from build123d import *

# Parameters (mm, degrees)
F1_DEPTH = 63.5
F2_DEPTH = 25.4


with BuildPart() as f1:
    # F0 (on Front) → F1 (new body, symmetric)
    with BuildSketch(Plane.XZ):
        Polygon((22.225, 9.525), (-41.275, 9.525), (-41.275, -9.525), (41.275, -9.525), (41.275, 9.525), align=None)
    extrude(amount=F1_DEPTH, both=True)

    # F0 (on Front) → F2 (join, symmetric)
    with BuildSketch(Plane.XZ):
        with BuildLine():
            add(Edge.make_bspline(
                [(-41.275, 9.525), (-17.963025, 64.389196), (-0.915335, 58.434684), (52.727391, 61.644047)],
                knots=[0, 0, 0, 0, 108.575172, 108.575172, 108.575172, 108.575172], degree=3))
            Line((-41.275, 9.525), (22.225, 9.525))
            Line((22.225, 9.525), (22.225, 27.0002))
            ThreePointArc((22.225, 27.0002), (30.937262, 50.079368), (52.727391, 61.644047))
        make_face()
        with BuildLine():
            Line((22.225, 27.0002), (22.225, 9.525))
            Line((22.225, 9.525), (41.275, 9.525))
            Line((41.275, 9.525), (41.275, 27.0002))
            ThreePointArc((41.275, 27.0002), (45.92468, 38.22552), (57.15, 42.8752))
            Line((57.15, 42.8752), (60.325, 42.8752))
            Line((60.325, 42.8752), (60.325, 61.9252))
            Line((60.325, 61.9252), (57.15, 61.9252))
            add(Edge.make_bspline(
                [(52.727391, 61.644047), (54.174675, 61.730636), (55.648598, 61.823896), (57.15, 61.9252)],
                knots=[108.575172, 108.575172, 108.575172, 108.575172, 111.504536, 111.504536, 111.504536, 111.504536], degree=3))
            ThreePointArc((52.727391, 61.644047), (30.937262, 50.079368), (22.225, 27.0002))
        make_face()
    extrude(amount=F2_DEPTH, both=True)


solid = f1.part
The listing builds one solid part. Answer for the finished solid, in the listing's coordinates (mm). A direction names the side the tool comes from. Coordinates: 2 decimals unless noted, no trailing zeros. Order: outer loops, then holes, each group sorted by start corner. A loop starts at its lowest first (then second) coordinate and runs counter-clockwise, first axis right, second up. Notation, with made-up numbers: (18.5, -20) -> (43.5, -20) arc R20 ccw to (43.5, -2) -> close; hole circle Ø7 at (27, 2.25). An arc over 180 degrees is marked (long way). Answer in a Markdown table with one row per item. Add a question column.
Item 1: Each of these flat-tipped pins is pushed along its axis until it touches: P1, Ø8, axis at x = 41.5, z = 21.5, coming from the -Y side; P2, Ø1, axis at y = -8, z = 12, coming from the -X side; P3, Ø12, axis at x = -8.5, z = 25, coming from the +Y side. Where does it stop, or does it pass through?
Item 2: Find the intervals of material crossed by L1, parallel to Y at x = 2.5, z = 26; L2, parallel to Z at x = 9, y = 35.5 (3 decimals); L3, parallel to X at y = 12.5, z = -5 (3 decimals), in increasing order. Write a range as from..to.
Item 3: Which of the six approach directions +Z, -Z, +X, -X, +Y, -Y give full straight-line access (tool end or side, diameter ignored) to faces 1 (the face through (1, -45, 9.525)), 2 (the face through (41.275, -1, 4)), 3 (the face through (-1, 63.5, 0)), 4 (the face through (1, 44, 9.525))?
Item 4: Find section A-A (z = -3.5). Write down the section's boundary in (x, y) (3 decimals), then the cut area to 3 significant figures.
Item 5: Find section B-B (y = 38). Write down the section's boundary in (x, z) (3 decimals), then the cut area to 3 significant figures.
Result set:
| question | item | result |
|---|---|---|
| 1 | P1 | stops at y = -25.4 |
| 1 | P2 | stops at x = -40.43 |
| 1 | P3 | stops at y = 25.4 |
| 2 | L1 | y = -25.4..25.4 |
| 2 | L2 | z = -9.525..9.525 |
| 2 | L3 | x = -41.275..41.275 |
| 3 | face 1 | +Z, +X, -X, -Y |
| 3 | face 2 | -Z, +X, +Y, -Y |
| 3 | face 3 | +Z, -Z, +X, -X, +Y |
| 3 | face 4 | +Z, +X, -X, +Y |
| 4 | outline | (-41.275, -63.5) -> (41.275, -63.5) -> (41.275, 63.5) -> (-41.275, 63.5) -> close |
| 4 | area | 10,500 mm² |
| 5 | outline | (-41.275, -9.525) -> (41.275, -9.525) -> (41.275, 9.525) -> (-41.275, 9.525) -> close |
| 5 | area | 1,570 mm² |
